from build123d import *

# Parameters (mm, degrees)
SKETCH1_R           = 2.1
BOSS_EXTRUDE1_DEPTH = 8
SKETCH2_R           = 3.2
CUT_EXTRUDE1_DEPTH  = 6
SKETCH3_R           = 2
CUT_EXTRUDE2_DEPTH  = 6
CHAMFER1_SIZE       = 1


with BuildPart() as part:
    # Sketch1 → Boss-Extrude1 (new body)
    with BuildSketch(Plane(origin=(0, 0, 0), x_dir=(1, 0, 0), z_dir=(0, 1, 0))):
        with BuildLine():
            Line((-14.7, 5), (14.7, 5))
            ThreePointArc((14.7, 5), (19.7, 0), (14.7, -5))
            Line((14.7, -5), (-14.7, -5))
            ThreePointArc((-14.7, -5), (-19.7, 0), (-14.7, 5))
        make_face()
        with Locations((-14.7, 0)):
            Circle(SKETCH1_R, mode=Mode.SUBTRACT)
        with Locations((14.7, 0)):
            Circle(SKETCH1_R, mode=Mode.SUBTRACT)
    extrude(amount=BOSS_EXTRUDE1_DEPTH)

    # Sketch2 → Cut-Extrude1 (cut)
    with BuildSketch(Plane(origin=(0, 8, 0), x_dir=(1, 0, 0), z_dir=(0, 1, 0))):
        Circle(SKETCH2_R)
    extrude(amount=-CUT_EXTRUDE1_DEPTH, mode=Mode.SUBTRACT)

    # Sketch3 → Cut-Extrude2 (cut)
    with BuildSketch(Plane.XZ):
        Circle(SKETCH3_R)
    extrude(amount=-CUT_EXTRUDE2_DEPTH, mode=Mode.SUBTRACT)

    # Chamfer1
    chamfer1_edges = [part.edges().sort_by_distance(p)[0] for p in [
        (-3.2, 8, 0),
    ]]
    chamfer(chamfer1_edges, length=CHAMFER1_SIZE)


solid = part.part
The listing builds one solid part. Answer for the finished solid, in the listing's coordinates (mm). A direction names the side the tool comes from. Coordinates: 2 decimals unless noted, no trailing zeros. Loops run counter-clockwise (first coordinate to the right, second up) from the corner with the lowest first, then second, coordinate; pieces in that order, holes last. Notation, with made-up numbers: M -39,-39.5 L 1,-39.5 A38 ccw 1,-1.5 Z; hole C 82,60 d6. An arc over 180 degrees is marked long. Answer in a Markdown table with one row per item.
1) Given pin 1 (3 mm diameter, centred on x = 0, z = 1.5, fed in from +Y); pin 2 (3 mm diameter, centred on x = 1.5, z = -1, fed in from +Y), each flat-ended and moving along its own axis, determine where each tip first touches the part or whether it passes through.
Answers below:
| item | result |
|---|---|
| pin 1 | y = 2 |
| pin 2 | y = 7.1 |
2) Find the intervals of material crossed by probe 1 along Z at (x, y) = (0, 0.6); probe 2 along Z at (x, y) = (0, 4.7); probe 3 along X at (y, z) = (4.3, 0), in increasing order.
Answers below:
| item | result |
|---|---|
| probe 1 | -5 to -2, 2 to 5 |
| probe 2 | -5 to -3.2, 3.2 to 5 |
| probe 3 | -19.7 to -16.8, -12.6 to -3.2, 3.2 to 12.6, 16.8 to 19.7 |
3) Which of the six approach directions +Z, -Z, +X, -X, +Y, -Y give full straight-line access (tool end or side, diameter ignored) to faces 4 (the flat face through (2, 2, 1)), 5 (the flat face through (0.3, 0, -2.3))?
Answers below:
| item | result |
|---|---|
| face 4 | +Y |
| face 5 | +Z, -Z, +X, -X, -Y |
4) Find section A-A (x = 0). Determine the outline of the cut face in (y, z).
Answers below:
| item | result |
|---|---|
| outline | M 0,-5 L 8,-5 L 8,-4.2 L 7,-3.2 L 2,-3.2 L 2,-2 L 0,-2 Z; M 0,2 L 2,2 L 2,3.2 L 7,3.2 L 8,4.2 L 8,5 L 0,5 Z |
5) Find section B-B (x = -16). Determine the outline of the cut face in (y, z).
Answers below:
| item | result |
|---|---|
| outline | M 0,-4.83 L 8,-4.83 L 8,-1.65 L 0,-1.65 Z; M 0,1.65 L 8,1.65 L 8,4.83 L 0,4.83 Z |
6) Find section C-C (x = 13). Determine the outline of the cut face in (y, z), then the cut area to 3 significant figures.
Answers below:
| item | result |
|---|---|
| outline | M 0,-5 L 8,-5 L 8,-1.23 L 0,-1.23 Z; M 0,1.23 L 8,1.23 L 8,5 L 0,5 Z |
| area | 60.3 mm^2 |
7) Determine the mould class of faces 1 (the cylindrical face through (-2.539, 4.535, 1.947)), 2 (the cylindrical face through (-19.7, 3.9, 0.1)), 3 (the flat face through (0.3, 8, 4.4)) for opening direction Z: released by +Z, released by -Z, zero draft, split by the parting line, or undercut.
Answers below:
| item | result |
|---|---|
| face 1 | undercut |
| face 2 | split by the parting line |
| face 3 | zero draft |
